```python
from build123d import *

# Parameters (mm, degrees)
BOSS_EXTRUDE1_DEPTH = 4.7
SKETCH2_OUTSIDE_W   = 42.786
SKETCH2_OUTSIDE_H   = 44.024
SKETCH2_OUTSIDE_R   = 4
CUT_EXTRUDE1_DEPTH  = 8.708653147
CUT_EXTRUDE1_DRAFT  = -60
SKETCH3_OUTSIDE_W   = 42.786
SKETCH3_OUTSIDE_H   = 44.024
SKETCH3_OUTSIDE_R   = 4
CUT_EXTRUDE2_DEPTH  = 8.708653147
CUT_EXTRUDE2_DRAFT  = -60
TAP1_D              = 4.134


with BuildPart() as part:
    # Sketch1 → Boss-Extrude1 (new body)
    with BuildSketch(Plane(origin=(0, 0, 0), x_dir=(0, 0, -1), z_dir=(1, 0, 0))):
        Polygon((0, 4.618802154), (-4, 2.309401077), (-4, -2.309401077), (0, -4.618802154), (4, -2.309401077), (4, 2.309401077), align=None)
    extrude(amount=-BOSS_EXTRUDE1_DEPTH)


with BuildPart() as cut_extrude1_tool:
    # Sketch2 outside → Cut-Extrude1 (with draft: the straight prism first)
    with BuildSketch(Plane(origin=(0, 0, 0), x_dir=(0, 0, -1), z_dir=(1, 0, 0))):
        Rectangle(SKETCH2_OUTSIDE_W, SKETCH2_OUTSIDE_H)
        Circle(SKETCH2_OUTSIDE_R, mode=Mode.SUBTRACT)
    extrude(amount=-CUT_EXTRUDE1_DEPTH)
    # Cut-Extrude1: the draft: its side faces are tilted about the plane it starts from
    cut_extrude1_sides = [cut_extrude1_tool.faces().sort_by_distance(p)[0] for p in [
        (-4.354326573, -22.012, 0),
        (-4.354326573, 0, -21.393),
        (-4.354326573, 22.012, 0),
        (-4.354326573, 0, 21.393),
        (-4.354326573, 0, 4),
    ]]
    draft(cut_extrude1_sides, Plane(origin=(0, 0, 0), x_dir=(0, 0, -1), z_dir=(1, 0, 0)), CUT_EXTRUDE1_DRAFT)


with BuildPart() as part_1:
    add(part.part)

    # Cut-Extrude1: cut by cut_extrude1_tool
    add(cut_extrude1_tool.part, mode=Mode.SUBTRACT)


with BuildPart() as cut_extrude2_tool:
    # Sketch3 outside → Cut-Extrude2 (with draft: the straight prism first)
    with BuildSketch(Plane.ZY.offset(4.7)):
        Rectangle(SKETCH3_OUTSIDE_W, SKETCH3_OUTSIDE_H)
        Circle(SKETCH3_OUTSIDE_R, mode=Mode.SUBTRACT)
    extrude(amount=-CUT_EXTRUDE2_DEPTH)
    # Cut-Extrude2: the draft: its side faces are tilted about the plane it starts from
    cut_extrude2_sides = [cut_extrude2_tool.faces().sort_by_distance(p)[0] for p in [
        (-0.345673427, -22.012, 0),
        (-0.345673427, 0, 21.393),
        (-0.345673427, 22.012, 0),
        (-0.345673427, 0, -21.393),
        (-0.345673427, 0, -4),
    ]]
    draft(cut_extrude2_sides, Plane.ZY.offset(4.7), CUT_EXTRUDE2_DRAFT)


with BuildPart() as part_2:
    add(part_1.part)

    # Cut-Extrude2: cut by cut_extrude2_tool
    add(cut_extrude2_tool.part, mode=Mode.SUBTRACT)

    # Tap1 (through all)
    with Locations(Plane(origin=(0, 0, 0), x_dir=(0, 0, -1), z_dir=(1, 0, 0))):
        with Locations((0, 0)):
            Hole(TAP1_D / 2)


solid = part_2.part
```
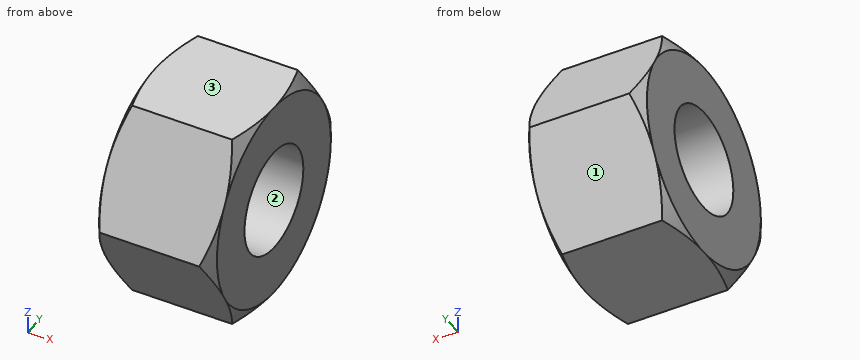
Design review of the part built by this model. Coordinates are the model's own, in mm. Face numbers are marked on the shaded views. Coordinates: 2 decimals unless noted, no trailing zeros. Order: outer loops, then holes, each group sorted by start corner. A loop starts at its lowest first (then second) coordinate and runs counter-clockwise, first axis right, second up.
1) Wall thickness on line 1 along Y through (x, z) = (-2.65, -1.5); line 2 along Z through (x, y) = (-3.8, 1.75); line 3 along Y through (x, z) = (-1.7, -0.75): over which ranges is each line inside the solid? List them lowest first.
2) Take a section at A-A, the plane x = -1.8. Give the boundary of the cut face in (y, z), and give its area (3 significant figures).
3) Mouldability with a two-part tool opening along Y and no side actions: class the marked faces 1, 2 and 3 as +Y half, -Y half, draft (parallel to the pull), parting line (faces both ways), or undercut.
Returned:
1. line 1: y = -3.75 to -1.42, 1.42 to 3.75
1. line 2: z = -4 to -1.1, 1.1 to 4
1. line 3: y = -4.19 to -1.93, 1.93 to 4.19
2. outline: (-4.62, 0) - (-2.31, -4) - (2.31, -4) - (4.62, 0) - (2.31, 4) - (-2.31, 4) - close; hole circle Ø4.13 at (0, 0)
2. area: 42.0 mm2
3. face 1: +Y half
3. face 2: undercut
3. face 3: draft
